from build123d import *

# Parameters (mm, degrees)
SKETCH_1_R      = 1.55
EXTRUDE_1_DEPTH = 2


with BuildPart() as part:
    # 草图1 → 凸台-拉伸1 (new body)
    with BuildSketch(Plane(origin=(0, 0, 0), x_dir=(1, 0, 0), z_dir=(0, 1, 0))):
        with BuildLine():
            Line((97.46, -4), (97.46, 52.29))
            ThreePointArc((97.46, 52.29), (96.874213562, 53.704213562), (95.46, 54.29))
            Line((95.46, 54.29), (-4, 54.29))
            ThreePointArc((-4, 54.29), (-5.414213562, 53.704213562), (-6, 52.29))
            Line((-6, 52.29), (-6, 17.45))
            Line((-6, 17.45), (-3.6, 17.45))
            Line((-3.6, 17.45), (-3.6, 9.75))
            Line((-3.6, 9.75), (-6, 9.75))
            Line((-6, 9.75), (-6, -4))
            ThreePointArc((-6, -4), (-5.414213562, -5.414213562), (-4, -6))
            Line((-4, -6), (95.46, -6))
            ThreePointArc((95.46, -6), (96.874213562, -5.414213562), (97.46, -4))
        make_face()
        Circle(SKETCH_1_R, mode=Mode.SUBTRACT)
        with Locations((91.46, 0)):
            Circle(SKETCH_1_R, mode=Mode.SUBTRACT)
        with Locations((0, 48.29)):
            Circle(SKETCH_1_R, mode=Mode.SUBTRACT)
        with Locations((91.46, 48.29)):
            Circle(SKETCH_1_R, mode=Mode.SUBTRACT)
    extrude(amount=EXTRUDE_1_DEPTH)


solid = part.part
Geometry: final body of the model. Coordinates: model frame, mm. A direction names the side the tool comes from. Give positions to 0.01 mm unless a question says otherwise; leave off trailing zeros. Write each loop counter-clockwise with the first axis right and the second up, starting at its lowest first coordinate (ties: lowest second). Pieces come first, ordered by that corner, then holes.
(1) Ray query, line 1 (Z direction, x = 91.46, y = 1.3); line 2 (X direction, y = 0.9, z = 0); line 3 (X direction, y = 0.2, z = -15). Return the intervals inside material, ascending.
(2) Mould query, pull axis X, two halves, no side actions, for faces 1 (the cylindrical face through (96.89, 0.99, -53.69)), 2 (the cylindrical face through (0.715, 0.986, 1.375)), 3 (the cylindrical face through (92.175, 0.986, -46.915)), 4 (the flat face through (-5, 1, -17.45)). Classes: released by +X, released by -X, zero draft, split by the parting line, or undercut.
(3) First-contact query: P1, Ø1, axis at x = -5, y = 0.5, coming from the +Z side; P2, Ø12, axis at x = 50.5, z = -1, coming from the -Y side; P3, Ø0.6, axis at x = -5, y = 1.5, coming from the -Z side. Flat tips, straight axial feed; report the tip coordinate or a pass-through.
(4) Cut plane A-A, the plane z = -48.29. Return loops of the section in (x, y).
(5) Cut plane B-B, the plane x = 0. Return loops of the section in (y, z), then the cut area to 3 significant figures.
(6) Access query for faces 5 (the flat face through (-3.6, 1, -14)), 6 (the cylindrical face through (96.86, 0.99, 5.43)). Directions: +Z, -Z, +X, -X, +Y, -Y. A direction counts if a zero-diameter tool reaches every point of the face in a straight line with its end or side. Return the directions, or none.
Values follow:
1. line 1: z = -54.29 to -49.84, -46.74 to -1.55, 1.55 to 6
1. line 2: x = -6 to -1.55, 1.55 to 89.91, 93.01 to 97.46
1. line 3: x = -3.6 to 97.46
2. face 1: released by +X
2. face 2: undercut
2. face 3: undercut
2. face 4: zero draft
3. P1: stops at z = 5.94
3. P2: stops at y = 0
3. P3: stops at z = -54.16
4. outline: (-6, 0) - (-1.55, 0) - (-1.55, 2) - (-6, 2) - close; (1.55, 0) - (89.91, 0) - (89.91, 2) - (1.55, 2) - close; (93.01, 0) - (97.46, 0) - (97.46, 2) - (93.01, 2) - close
5. outline: (0, -54.29) - (2, -54.29) - (2, -49.84) - (0, -49.84) - close; (0, -46.74) - (2, -46.74) - (2, -1.55) - (0, -1.55) - close; (0, 1.55) - (2, 1.55) - (2, 6) - (0, 6) - close
5. area: 108 mm2
6. face 5: -X, +Y, -Y
6. face 6: +Z, +X, +Y, -Y
